Autodesk Inventor part; units mm, degrees
ref_plane "YZ Plane" through (0, 0, 0) normal (1, 0, 0) x (0, 1, 0)
ref_plane "XZ Plane" through (0, 0, 0) normal (0, 1, 0) x (-1, 0, 0)
ref_plane "XY Plane" through (0, 0, 0) normal (0, 0, 1) x (1, 0, 0)
sketch "Esboço1" plane through (0, 0, 0) normal (1, 0, 0) x (0, 1, 0)
  line L0 (0, 0) -> (64.55, 0)
  line L1 (64.55, 0) -> (64.55, 3)
  line L2 (64.55, 55) -> (64.55, 58)
  line L3 (64.55, 58) -> (0, 58)
  line L4 (0, 58) -> (0, 0)
  line L5 (0, 58) -> (0, 55)
  line L6 (2, 55) -> (2, 3)
  line L7 (2, 3) -> (64.55, 3)
  line L8 (2, 55) -> (64.55, 55)
  dimension "d6" = 64.55
  dimension "d7" = 58
  dimension "d81" = 64.55
  dimension "d83" = 2
  dimension "d84" = 52
  dimension "d85" = 62.55
  dimension "d86" = 62.55
  dimension "d111" = 3
  dimension "d112" = 3
extrude "Extrusão1" add sketch "Esboço1" along normal blind 25
sketch "Esboço2" plane through (0, 0, 58) normal (0, 0, 1) x (1, 0, 0)
  line L0 (0, 0) -> (25, 0)
  circle A0 centre (12.5, 14.4) radius 1.75
  circle A1 centre (12.5, 51.85) radius 4.1
  circle A2 centre (12.5, 45.05) radius 1.75
  line L1 (12.5, 51.85) -> (16.5, 51.85) construction
  line L2 (12.5, 51.85) -> (19.3, 51.85) construction
  circle A3 centre (7.691674, 47.041674) radius 1.25
  circle A4 centre (19.3, 51.85) radius 1.75
  circle A5 centre (12.5, 58.65) radius 1.75
  circle A6 centre (5.7, 51.85) radius 1.75
  circle A7 centre (17.308326, 47.041674) radius 1.25
  circle A8 centre (17.308326, 56.658326) radius 1.25
  circle A9 centre (7.691674, 56.658326) radius 1.25
  line L3 (0, 0) -> (25, 0)
  line L4 (25, 2) -> (25, 64.55)
  line L5 (0, 31) -> (0, 64.55)
  line L6 (0, 64.55) -> (25, 64.55)
  line L7 (25, 64.55) -> (25, 31)
  circle A10 centre (12.5, 33) radius 1.75
  line L8 (29.4167, 51.85) -> (-4.4167, 51.85)
  arc A11 (25, 51.85) -> (0, 51.85) centre (12.5, 52.048425) ccw
  point P0 (12.5, 0)
  point P1 (12.5, 64.55)
  point P2 (12.5, 0)
  point P3 (12.5, 0)
  point P4 (0, 52.24685)
  point P5 (25, 52.24685)
  dimension "d11" = 3.5
  dimension "d42" = 2.5
  dimension "d53" = 360
  dimension "d59" = 360
  dimension "d88" = 12.7
  dimension "d89" = 14.4
  dimension "d94" = 3.5
  dimension "d95" = 33
  dimension "d113" = 3.5
  dimension "d114" = 8.2
sketch "Esboço2 outline for Extrusão2" plane through (0, 0, 58) normal (0, 0, 1) x (1, 0, 0)
  circle A0 centre (12.5, 14.4) radius 1.75
  circle A1 centre (12.5, 51.85) radius 4.1
  circle A2 centre (12.5, 45.05) radius 1.75
  circle A3 centre (7.691674, 47.041674) radius 1.25
  circle A4 centre (17.308326, 47.041674) radius 1.25
  circle A5 centre (17.308326, 56.658326) radius 1.25
  circle A6 centre (12.5, 58.65) radius 1.75
  circle A7 centre (5.7, 51.85) radius 1.75
  circle A8 centre (7.691674, 56.658326) radius 1.25
  circle A9 centre (19.3, 51.85) radius 1.75
  circle A10 centre (12.5, 33) radius 1.75
  arc A11 (0, 52.24685) -> (12.5, 64.55) centre (12.5, 52.048425) cw
  line L0 (0, 64.55) -> (0, 52.24685)
  line L1 (12.5, 64.55) -> (0, 64.55)
  arc A12 (12.5, 64.55) -> (25, 52.24685) centre (12.5, 52.048425) cw
  line L2 (25, 64.55) -> (12.5, 64.55)
  line L3 (25, 52.24685) -> (25, 64.55)
extrude "Extrusão2" cut sketch "Esboço2 outline for Extrusão2" against normal through all
sketch "Esboço4" plane through (0, 0, 0) normal (0, -1, 0) x (1, 0, 0)
  line L0 (0, 58) -> (25, 58)
  line L1 (14.25, 0) -> (10.75, 0)
  line L2 (25, 2) -> (25, 54)
  line L3 (0, 2) -> (0, 54)
  circle A0 centre (12.5, 29) radius 4.1
  circle A1 centre (12.583333, 22) radius 1.75
  line L4 (12.5, 29) -> (16.5, 29) construction
  line L5 (12.5, 29) -> (19.3, 29) construction
  circle A2 centre (7.357232, 23.889772) radius 1.25
  circle A3 centre (19.5, 29.083333) radius 1.75
  circle A4 centre (12.416667, 36) radius 1.75
  circle A5 centre (5.5, 28.916667) radius 1.75
  circle A6 centre (17.610228, 23.857232) radius 1.25
  circle A7 centre (17.642768, 34.110228) radius 1.25
  circle A8 centre (7.389772, 34.142768) radius 1.25
  line L6 (0, 0) -> (25, 0)
  circle A9 centre (12.5, 47) radius 1.75
  circle A10 centre (12.5, 11) radius 1.75
  line L7 (25, 0) -> (25, 1)
  line L8 (25, 58) -> (25, 0)
  line L9 (25, 58) -> (25, 57)
  line L10 (25, 57) -> (25, 2)
  line L11 (12.5, 0) -> (12.5, 58)
  point P0 (24.956484, 28.030424)
  dimension "d68" = 8.2
  dimension "d69" = 3.5
  dimension "d70" = 2.5
  dimension "d72" = 360
  dimension "d74" = 360
  dimension "d97" = 29
  dimension "d109" = 3.5
  dimension "d110" = 3.5
  dimension "d118" = 11
  dimension "d124" = 11
  dimension "d125" = 5.5
  dimension "d126" = 5.5
  dimension "d127" = 12.5
  dimension "d128" = 12.5
  dimension "d129" = 12.5
  dimension "d130" = 12.5
extrude "Extrusão3" cut sketch "Esboço4" against normal through all contours L11 A9 | A9 L11 | L11 A4 | A4 L11 | L11 A0 | A0 L11 | L11 A1 | A1 L11 | L11 A10 | A10 L11 | A2 | A3 | A5 | A6 | A7 | A8
fillet "Arredondamento1" radius 2 2 edges at (12.5, 0, 0) (12.5, 0, 58)
chamfer "Chanfro1" distance 2 angle 45 2 edges at (12.5, 2, 55) (12.5, 2, 3)
properties part number "long FrameARRUMADO"
Input: part model. Units: mm. Frame: model coordinates. A direction names the side the tool comes from. Round coordinates to 2 decimals unless told otherwise and drop trailing zeros. Loops run counter-clockwise (first coordinate to the right, second up) from the corner with the lowest first, then second, coordinate; pieces in that order, holes last. Notation, with made-up numbers: (89, 33) -> (134, 33) arc R26 ccw to (134, 62) -> close; hole circle Ø2 at (29.5, 26). An arc over 180 degrees is marked (long way). Answer as a JSON object with one key per item and string values. Group by question number.
1) Reachability of faces 1 (the flat face through (15, 34, 3)), 2 (the cylindrical face through (14.169, 45.576, 1.521)) from +Z, -Z, +X, -X, +Y, -Y: full face, straight path, thin tool, end or side. Return the list, or none.
2) Ray query, L1, parallel to Z at x = 1.5, y = 41.5; L2, parallel to X at y = 45, z = 56; L3, parallel to Y at x = 11.25, z = 18.5. Return the intervals inside material, ascending.
3) Pin query (flat end, axial travel): pin 1 (1.5 mm diameter, centred on x = 10, z = 14, fed in from -Y); pin 2 (5.5 mm diameter, centred on x = 12.5, z = 47, fed in from +Y). Return the tip coordinate at first contact, or that it passes through.
4) Section query C-C on x = 20. Output: boundary loops of the cut face in (y, z), plus the area to 3 significant figures.
5) Draft query along X for faces 3 (the flat face through (25, 1, 29)), 4 (the cylindrical face through (12.68, 0.6, 57.43)), 5 (the flat face through (0, 1, 29)), 6 (the cylindrical face through (18.463, 56.18, 56.521)). Return one class per face: +X half, -X half, draft (parallel to the pull), parting line (faces both ways), or undercut.
6) Section query B-B on z = 47. Output: boundary loops of the cut face in (x, y), plus the area to 3 significant figures.
7) Section query D-D on z = 7. Output: boundary loops of the cut face in (x, y), plus the area to 3 significant figures.
8) Section query A-A on y = 45.05. Output: boundary loops of the cut face in (x, z), plus the area to 3 significant figures.
Reply:
{
 "1": {"face 1": "+X, -X, +Y", "face 2": "+Z, -Z"},
 "2": {"L1": "z = 0 to 3, 55 to 58", "L2": "x = 0 to 10.75, 14.25 to 25", "L3": "y = 0 to 2"},
 "3": {"pin 1": "stops at y = 0", "pin 2": "stops at y = 2"},
 "4": {"outline": "(0, 2) arc R2 ccw to (2, 0) -> (50.25, 0) -> (50.25, 3) -> (4, 3) -> (2, 5) -> (2, 27.41) -> (0, 27.41) -> close; (0, 30.76) -> (2, 30.76) -> (2, 53) -> (4, 55) -> (50.25, 55) -> (50.25, 58) -> (2, 58) arc R2 ccw to (0, 56) -> close; (53.45, 0) -> (62.05, 0) -> (62.05, 3) -> (53.45, 3) -> close; (53.45, 55) -> (62.05, 55) -> (62.05, 58) -> (53.45, 58) -> close", "area": "453 mm2"},
 "5": {"face 3": "+X half", "face 4": "draft", "face 5": "-X half", "face 6": "undercut"},
 "6": {"outline": "(0, 0) -> (10.75, 0) -> (10.75, 2) -> (0, 2) -> close; (14.25, 0) -> (25, 0) -> (25, 2) -> (14.25, 2) -> close", "area": "43.0 mm2"},
 "7": {"outline": "(0, 0) -> (25, 0) -> (25, 2) -> (0, 2) -> close", "area": "50.0 mm2"},
 "8": {"outline": "(0, 0) -> (10.75, 0) -> (10.75, 3) -> (0, 3) -> close; (0, 55) -> (10.75, 55) -> (10.75, 58) -> (0, 58) -> close; (14.25, 0) -> (25, 0) -> (25, 3) -> (14.25, 3) -> close; (14.25, 55) -> (25, 55) -> (25, 58) -> (14.25, 58) -> close", "area": "129 mm2"}
}
